from build123d import *

# Parameters (mm, degrees)
F1_R     = 2.45
F2_DEPTH = 10
F3_DEPTH = 5
F5_DEPTH = 2


with BuildPart() as f2:
    # F1 (on Front) → F2 (new body)
    with BuildSketch(Plane.XZ):
        with Locations((-43, 24)):
            Circle(F1_R)
        with Locations((-43, -24)):
            Circle(F1_R)
        with Locations((43, -24)):
            Circle(F1_R)
        with Locations((43, 24)):
            Circle(F1_R)
    extrude(amount=F2_DEPTH)



with BuildPart() as f3:
    # F0 (on Front) → F3 (new body)
    with BuildSketch(Plane.XZ):
        with BuildLine():
            ThreePointArc((49, 24), (47.242641, 28.242641), (43, 30))
            Line((43, 30), (-43, 30))
            ThreePointArc((-43, 30), (-47.242641, 28.242641), (-49, 24))
            Line((-49, 24), (-49, -24))
            ThreePointArc((-49, -24), (-47.242641, -28.242641), (-43, -30))
            Line((-43, -30), (43, -30))
            ThreePointArc((43, -30), (47.242641, -28.242641), (49, -24))
            Line((49, -24), (49, 24))
        make_face()
        with BuildLine():
            ThreePointArc((47, -24), (45.828427, -26.828427), (43, -28))
            Line((43, -28), (-43, -28))
            ThreePointArc((-43, -28), (-45.828427, -26.828427), (-47, -24))
            Line((-47, -24), (-47, 24))
            ThreePointArc((-47, 24), (-45.828427, 26.828427), (-43, 28))
            Line((-43, 28), (43, 28))
            ThreePointArc((43, 28), (45.828427, 26.828427), (47, 24))
            Line((47, 24), (47, -24))
        make_face(mode=Mode.SUBTRACT)
    extrude(amount=F3_DEPTH)


with BuildPart() as f2_1:
    add(f2.part)

    add(f3.part)  # F5 merges F3
    # F4 (on face) → F5 (join)
    with BuildSketch(Plane(origin=(0, 0, 0), x_dir=(-1, 0, 0), z_dir=(0, 1, 0))):
        with BuildLine():
            Line((43.864976, 30), (-43.864976, 30))
            ThreePointArc((-43.864976, 30), (-47.400509, 28.535534), (-48.864976, 25))
            Line((-48.864976, 25), (-48.864976, -25))
            ThreePointArc((-48.864976, -25), (-47.400509, -28.535534), (-43.864976, -30))
            Line((-43.864976, -30), (43.864976, -30))
            ThreePointArc((43.864976, -30), (47.400509, -28.535534), (48.864976, -25))
            Line((48.864976, -25), (48.864976, 25))
            ThreePointArc((48.864976, 25), (47.400509, 28.535534), (43.864976, 30))
        make_face()
    extrude(amount=F5_DEPTH)


solid = f2_1.part
Here's how the part is built. I have some questions about the finished solid (model axes, mm). A direction names the side the tool comes from. Coordinates: 2 decimals unless noted, no trailing zeros. Write each loop counter-clockwise with the first axis right and the second up, starting at its lowest first coordinate (ties: lowest second). Pieces come first, ordered by that corner, then holes.
Item 1: If I drill on line 1 (Z direction, x = -27.5, y = -3); line 2 (X direction, y = -1.25, z = 4); line 3 (Y direction, x = 23, z = -10), over which ranges is the centre line in solid material (lowest first)?
Item 2: I want a section at D-D on y = -8.5. Write out the boundary of the cut face in (x, z), and give its area (3 significant figures).
Item 3: I want a section at B-B on x = 11. Write out the boundary of the cut face in (y, z).
Item 4: If we mould it in two halves opening along Z, with no side actions, what happens to faces 1 (the flat face through (-43, -10, -24)), 2 (the cylindrical face through (45.859, -2.465, -26.797)), 3 (the cylindrical face through (47.196, -2.465, -28.289)), 4 (the cylindrical face through (-45.859, -2.465, 26.797))? For each: +Z half, -Z half, draft (parallel to the pull), parting line (faces both ways), or undercut.
Item 5: On a 3-axis mill with a long thin cutter (end or side, diameter ignored), from which of +Z, -Z, +X, -X, +Y, -Y can I reach the whole of each face in a straight line? I mean faces 5 (the cylindrical face through (-40.663, -4.93, 24.736)), 6 (the flat face through (-47, 0, -28.7)), 7 (the flat face through (47, 0, -28.7)), 8 (the flat face through (-47, 0, 28.7)), 9 (the flat face through (-48.865, 1, 0)). Say none if no direction works.
Item 6: I want a section at A-A on y = -3. Write out the boundary of the cut face in (x, z), and give its area (3 significant figures).
Item 7: Will these pins go through, and if not, where does the flat tip stop? pin 1 (3 mm diameter, centred on x = -23.5, z = 19.5, fed in from -Y); pin 2 (2.5 mm diameter, centred on x = -47, z = -27.5, fed in from -Y); pin 3 (1.6 mm diameter, centred on y = 1, z = 7.5, fed in from +X) (3 decimals).
Item 8: I want a section at C-C on z = -4. Write out the boundary of the cut face in (x, y), and give its area (3 significant figures).
Findings below:
1. line 1: z = -30 to -28, 28 to 30
1. line 2: x = -49 to -47, 47 to 49
1. line 3: y = 0 to 2
2. outline: circle Ø4.9 at (-43, -24); circle Ø4.9 at (-43, 24); circle Ø4.9 at (43, -24); circle Ø4.9 at (43, 24)
2. area: 75.4 mm2
3. outline: (-5, -30) - (2, -30) - (2, 30) - (-5, 30) - (-5, 28) - (0, 28) - (0, -28) - (-5, -28) - close
4. face 1: draft
4. face 2: undercut
4. face 3: -Z half
4. face 4: undercut
5. face 5: -Y
5. face 6: -Z, -X, -Y
5. face 7: -Z, +X, -Y
5. face 8: +Z, -X, -Y
5. face 9: +Z, -Z, -X, +Y
6. outline: (-49, -24) arc R6 ccw to (-43, -30) - (43, -30) arc R6 ccw to (49, -24) - (49, 24) arc R6 ccw to (43, 30) - (-43, 30) arc R6 ccw to (-49, 24) - close; circle Ø4.9 at (-43, -24); circle Ø4.9 at (-43, 24); circle Ø4.9 at (43, -24); circle Ø4.9 at (43, 24); hole (-47, -24) arc R4 ccw to (-43, -28) - (43, -28) arc R4 ccw to (47, -24) - (47, 24) arc R4 ccw to (43, 28) - (-43, 28) arc R4 ccw to (-47, 24) - close
6. area: 674 mm2
7. pin 1: stops at y = 0
7. pin 2: stops at y = -5
7. pin 3: stops at x = 48.865
8. outline: (-49, -5) - (-47, -5) - (-47, 0) - (47, 0) - (47, -5) - (49, -5) - (49, 0) - (48.86, 0) - (48.86, 2) - (-48.86, 2) - (-48.86, 0) - (-49, 0) - close
8. area: 215 mm2
